Design review of the part built by this model. Coordinates are the model's own, in mm. A direction names the side the tool comes from. Give positions to 0.01 mm unless a question says otherwise; leave off trailing zeros. Order: outer loops, then holes, each group sorted by start corner. A loop starts at its lowest first (then second) coordinate and runs counter-clockwise, first axis right, second up. Notation, with made-up numbers: (79.5, 10) -> (136.5, 10) arc R29 cw to (136.5, 47) -> close; hole circle Ø4 at (2.5, -40). An arc over 180 degrees is marked (long way). One line per item, written item: value. Start each with the question number.
1) The part is to be moulded in two halves that separate along X. For faces 4 (the face through (12.75, 2, 2)), 5 (the face through (-12.134, 4.849, 1.972)), 6 (the face through (5.7, 19.5, 2)), say which applies: released by +X, released by -X, zero draft, split by the parting line, or undercut.
2) Consider section B-B (y = 36.5). State the section outline as (x, z) points, plus the area to 3 significant figures.
3) Consider section D-D (x = 6.5). State the section outline as (y, z) points, plus the area to 3 significant figures.
4) Tool access review of faces 1 (the face through (12.116, 4.901, 1.972)), 2 (the face through (0, 0, 2)), 3 (the face through (-7, 21, 2)): name each direction out of +Z, -Z, +X, -X, +Y, -Y from which nothing blocks a thin tool from reaching the whole face with its end or side.
5) For pin 1 (1.5 mm diameter, centred on y = 2, z = 2, fed in from -X); pin 2 (1.2 mm diameter, centred on y = 12.5, z = 1, fed in from +X); pin 3 (1.5 mm diameter, centred on y = 2, z = 2, fed in from +X), all flat-tipped, find the tip position at first contact; note any pin that passes through.
6) Consider section A-A (x = 0). State the section outline as (y, z) points, plus the area to 3 significant figures.
7) Wall thickness on line 1 along X through (y, z) = (9.5, 1.95); line 2 along Y through (x, z) = (0, 1.75); line 3 along X through (y, z) = (36.5, 2.95): over which ranges is each line inside the solid? List them lowest first. Write a range as from..to.
8) Consider section C-C (z = 1.25). State the section outline as (x, y) points, plus the area to 3 significant figures.
from build123d import *

# Parameters (mm, degrees)
DODANIE_WYCI_GNI_CIE1_DEPTH = 4


with BuildPart() as part:
    # Szkic1 → Dodanie-wyciągnięcie1 (new body)
    with BuildSketch(Plane.XY):
        with BuildLine():
            Line((12.75, 0), (-12.75, 0))
            Line((-12.75, 0), (-12.75, 3))
            Line((-12.75, 3), (-11.5, 6.75))
            Line((-11.5, 6.75), (-11.5, 26.107695155))
            ThreePointArc((-11.5, 26.107695155), (0, 52), (11.5, 26.107695155))
            Line((11.5, 26.107695155), (11.5, 6.75))
            Line((11.5, 6.75), (12.75, 3))
            Line((12.75, 3), (12.75, 0))
        make_face()
        with BuildLine():
            Line((-2, 14.15), (-2, 9.15))
            ThreePointArc((-2, 9.15), (-5.25, 5.9), (-8.5, 9.15))
            Line((-8.5, 9.15), (-8.5, 14.15))
            Line((-8.5, 14.15), (-8.5, 25.375702269))
            ThreePointArc((-8.5, 25.375702269), (7.766114148, 48.148496514), (-7, 24.375644347))
            Line((-7, 24.375644347), (-7, 16.888612788))
            ThreePointArc((-7, 16.888612788), (-3.6887505, 17.000438563), (-2, 14.15))
        make_face(mode=Mode.SUBTRACT)
        with BuildLine():
            Line((9, 16.25), (9, 8.25))
            ThreePointArc((9, 8.25), (5.75, 5), (2.5, 8.25))
            Line((2.5, 8.25), (2.5, 16.25))
            ThreePointArc((2.5, 16.25), (5.75, 19.5), (9, 16.25))
        make_face(mode=Mode.SUBTRACT)
    extrude(amount=DODANIE_WYCI_GNI_CIE1_DEPTH)


solid = part.part
Checked values:
1. face 4: released by +X
1. face 5: released by -X
1. face 6: undercut
2. outline: (-15.5, 0) -> (-14, 0) -> (-14, 4) -> (-15.5, 4) -> close; (14, 0) -> (15.5, 0) -> (15.5, 4) -> (14, 4) -> close
2. area: 12.0 mm^2
3. outline: (0, 0) -> (5.09, 0) -> (5.09, 4) -> (0, 4) -> close; (19.41, 0) -> (24.1, 0) -> (24.1, 4) -> (19.41, 4) -> close; (48.9, 0) -> (50.57, 0) -> (50.57, 4) -> (48.9, 4) -> close
3. area: 45.8 mm^2
4. face 1: +Z, -Z, +X
4. face 2: +Z, -Z, +X, -X, -Y
4. face 3: +Z, -Z
5. pin 1: stops at x = -12.75
5. pin 2: stops at x = 11.5
5. pin 3: stops at x = 12.75
6. outline: (0, 0) -> (22.5, 0) -> (22.5, 4) -> (0, 4) -> close; (50.5, 0) -> (52, 0) -> (52, 4) -> (50.5, 4) -> close
6. area: 96.0 mm^2
7. line 1: x = -11.5..-8.5, -2..2.5, 9..11.5
7. line 2: y = 0..22.5, 50.5..52
7. line 3: x = -15.5..-14, 14..15.5
8. outline: (-12.75, 0) -> (12.75, 0) -> (12.75, 3) -> (11.5, 6.75) -> (11.5, 26.11) arc R15.5 ccw (long way) to (-11.5, 26.11) -> (-11.5, 6.75) -> (-12.75, 3) -> close; hole (-8.5, 9.15) arc R3.25 ccw to (-2, 9.15) -> (-2, 14.15) arc R3.25 ccw to (-7, 16.89) -> (-7, 24.38) arc R14 ccw (long way) to (-8.5, 25.38) -> close; hole (2.5, 8.25) arc R3.25 ccw to (9, 8.25) -> (9, 16.25) arc R3.25 ccw to (2.5, 16.25) -> close
8. area: 506 mm^2
